from build123d import *

# Parameters (mm, degrees)
SKETCH1_W           = 258
SKETCH1_H           = 40
SKETCH1_R           = 2.5
BOSS_EXTRUDE1_DEPTH = 4


with BuildPart() as part:
    # Sketch1 → Boss-Extrude1 (new body)
    with BuildSketch(Plane.XY):
        Rectangle(SKETCH1_W, SKETCH1_H)
        with Locations((-69.5, 10)):
            Circle(SKETCH1_R, mode=Mode.SUBTRACT)
        with Locations((-19.5, 10)):
            Circle(SKETCH1_R, mode=Mode.SUBTRACT)
        with Locations(Location((17, 10, 0), (0, 0, 180))):
            Circle(SKETCH1_R, mode=Mode.SUBTRACT)
        with Locations(Location((67, 10, 0), (0, 0, 180))):
            Circle(SKETCH1_R, mode=Mode.SUBTRACT)
        with Locations((-69.5, -7)):
            Circle(SKETCH1_R, mode=Mode.SUBTRACT)
        with Locations((-19.5, -7)):
            Circle(SKETCH1_R, mode=Mode.SUBTRACT)
        with Locations(Location((17, -7, 0), (0, 0, 180))):
            Circle(SKETCH1_R, mode=Mode.SUBTRACT)
        with Locations(Location((67, -7, 0), (0, 0, 180))):
            Circle(SKETCH1_R, mode=Mode.SUBTRACT)
    extrude(amount=BOSS_EXTRUDE1_DEPTH)


solid = part.part
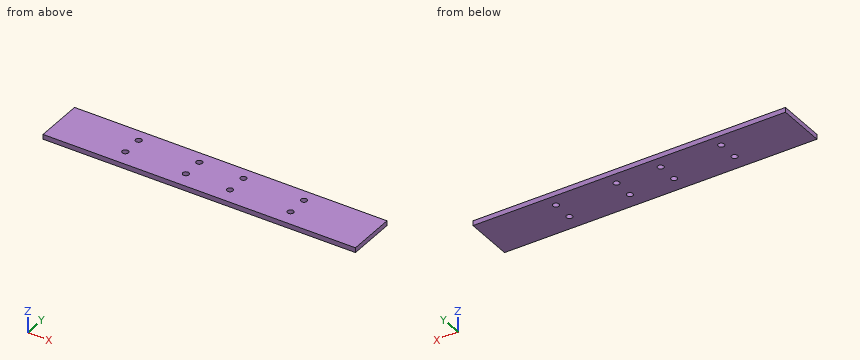
Can you work these out from the model? Positions are in its coordinate system, mm. Coordinates: 2 decimals unless noted, no trailing zeros. Write each loop counter-clockwise with the first axis right and the second up, starting at its lowest first coordinate (ties: lowest second). Pieces come first, ordered by that corner, then holes. Notation, with made-up numbers: (71.25, -32.5) -> (121.25, -32.5) arc R23 ccw to (121.25, -11.5) -> close; hole circle Ø9 at (51, 58.5). An arc over 180 degrees is marked (long way). Write each question's results on one line, items separated by ' | '. Start each with the question number.
Item 1: If we section it at A-A, the plane z = 2.9: Count the separate pieces of the cut face and the enclosed holes in it, and give its area (3 significant figures).
Item 2: If we section it at C-C, the plane y = 10: Write out the boundary of the cut face in (x, z), and give its area (3 significant figures).
Item 3: If we section it at B-B, the plane x = -19.5: Write out the boundary of the cut face in (y, z).
Item 4: Please list where these lines run through material, in increasing order: probe 1 along Y at (x, z) = (17, 1.55); probe 2 along X at (y, z) = (11, 0.4); probe 3 along X at (y, z) = (-9, 3.5).
Answer block:
1) separate pieces: 1 | enclosed holes: 8 | area: 10,200 mm²
2) outline: (-129, 0) -> (-72, 0) -> (-72, 4) -> (-129, 4) -> close; (-67, 0) -> (-22, 0) -> (-22, 4) -> (-67, 4) -> close; (-17, 0) -> (14.5, 0) -> (14.5, 4) -> (-17, 4) -> close; (19.5, 0) -> (64.5, 0) -> (64.5, 4) -> (19.5, 4) -> close; (69.5, 0) -> (129, 0) -> (129, 4) -> (69.5, 4) -> close | area: 952 mm²
3) outline: (-20, 0) -> (-9.5, 0) -> (-9.5, 4) -> (-20, 4) -> close; (-4.5, 0) -> (7.5, 0) -> (7.5, 4) -> (-4.5, 4) -> close; (12.5, 0) -> (20, 0) -> (20, 4) -> (12.5, 4) -> close
4) probe 1: -20 to -9.5, -4.5 to 7.5, 12.5 to 20 | probe 2: -129 to -71.79, -67.21 to -21.79, -17.21 to 14.71, 19.29 to 64.71, 69.29 to 129 | probe 3: -129 to -71, -68 to -21, -18 to 15.5, 18.5 to 65.5, 68.5 to 129
